Print and shaded views of the part. All mm, measured from the part's lowest x, y and z. A direction names the side the tool comes from. Give positions to 0.01 mm unless a question says otherwise; leave off trailing zeros. Write each loop counter-clockwise with the first axis right and the second up, starting at its lowest first coordinate (ties: lowest second). Pieces come first, ordered by that corner, then holes.
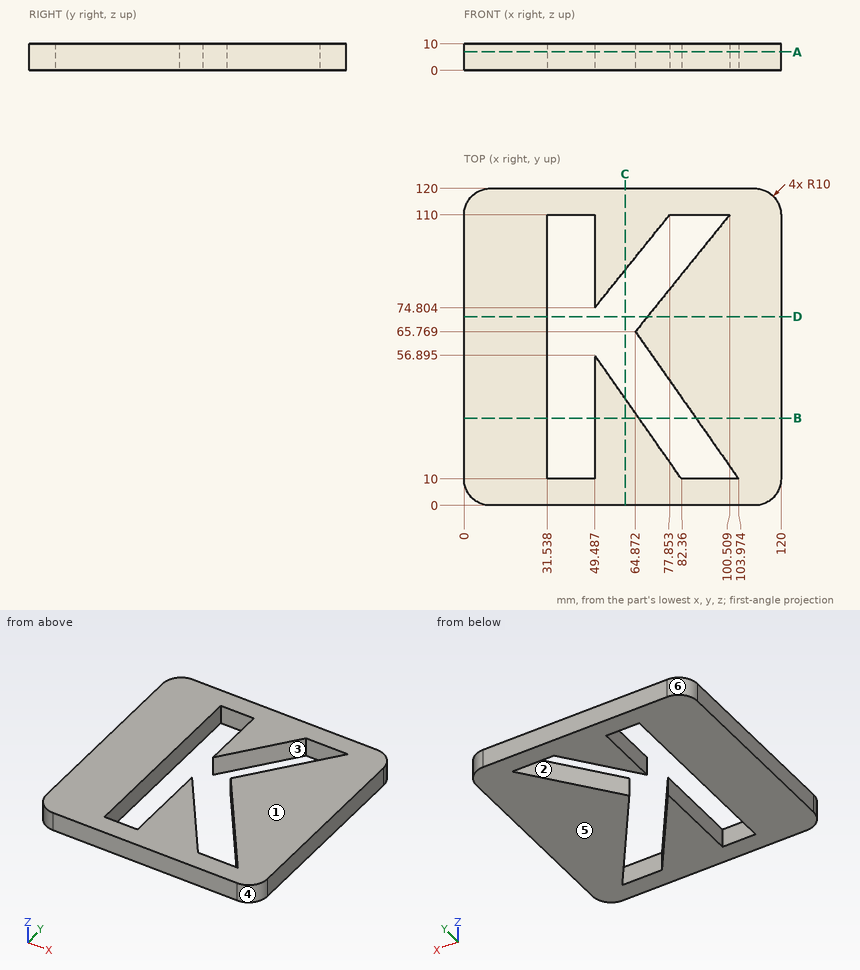
1. Saw through at B-B on y = 33. Give the cut face in (x, z).
2. Saw through at A-A on z = 7. Give the cut face in (x, y) (1 decimal), plus the area to 3 significant figures.
3. Saw through at D-D on y = 71.5. Give the cut face in (x, z).
4. 3-axis set-ups, long thin cutter, end or side, ignore diameter. For the marked faces 1 and 2: which of +Z, -Z, +X, -X, +Y, -Y reach the whole face in a straight line?
5. Drill centre lines: line 1 along Y through (x, z) = (39, 4); line 2 along X through (y, z) = (35, 6.5) (1 decimal); line 3 along X through (y, z) = (84.5, 5) (1 decimal). Where is each one in solid material? Low to high.
6. Mould opens along Y. For the marked faces 3, 4, 5 and 6 say: pulls with the +Y half, pulls with the -Y half, needs draft (parallel to the pull), parting line crosses it, or undercut.
7. Saw through at C-C on x = 61. Give the cut face in (y, z), plus the area to 3 significant figures.
Outcome:
1. outline: (0, 0) - (31.54, 0) - (31.54, 10) - (0, 10) - close; (49.49, 0) - (66.24, 0) - (66.24, 10) - (49.49, 10) - close; (87.85, 0) - (120, 0) - (120, 10) - (87.85, 10) - close
2. outline: (0, 10) arc R10 ccw to (10, 0) - (110, 0) arc R10 ccw to (120, 10) - (120, 110) arc R10 ccw to (110, 120) - (10, 120) arc R10 ccw to (0, 110) - close; hole (31.5, 10) - (49.5, 10) - (49.5, 56.9) - (82.4, 10) - (104, 10) - (64.9, 65.8) - (100.5, 110) - (77.9, 110) - (49.5, 74.8) - (49.5, 110) - (31.5, 110) - close
2. area: 10,400 mm2
3. outline: (0, 0) - (31.54, 0) - (31.54, 10) - (0, 10) - close; (69.49, 0) - (120, 0) - (120, 10) - (69.49, 10) - close
4. face 1: +Z, +X, -X, +Y, -Y
4. face 2: +Z, -Z
5. line 1: y = 0 to 10, 110 to 120
5. line 2: x = 0 to 31.5, 49.5 to 64.8, 86.4 to 120
5. line 3: x = 0 to 31.5, 49.5 to 57.3, 80 to 120
6. face 3: undercut
6. face 4: pulls with the -Y half
6. face 5: needs draft
6. face 6: pulls with the +Y half
7. outline: (0, 0) - (40.47, 0) - (40.47, 10) - (0, 10) - close; (89.09, 0) - (120, 0) - (120, 10) - (89.09, 10) - close
7. area: 714 mm2
